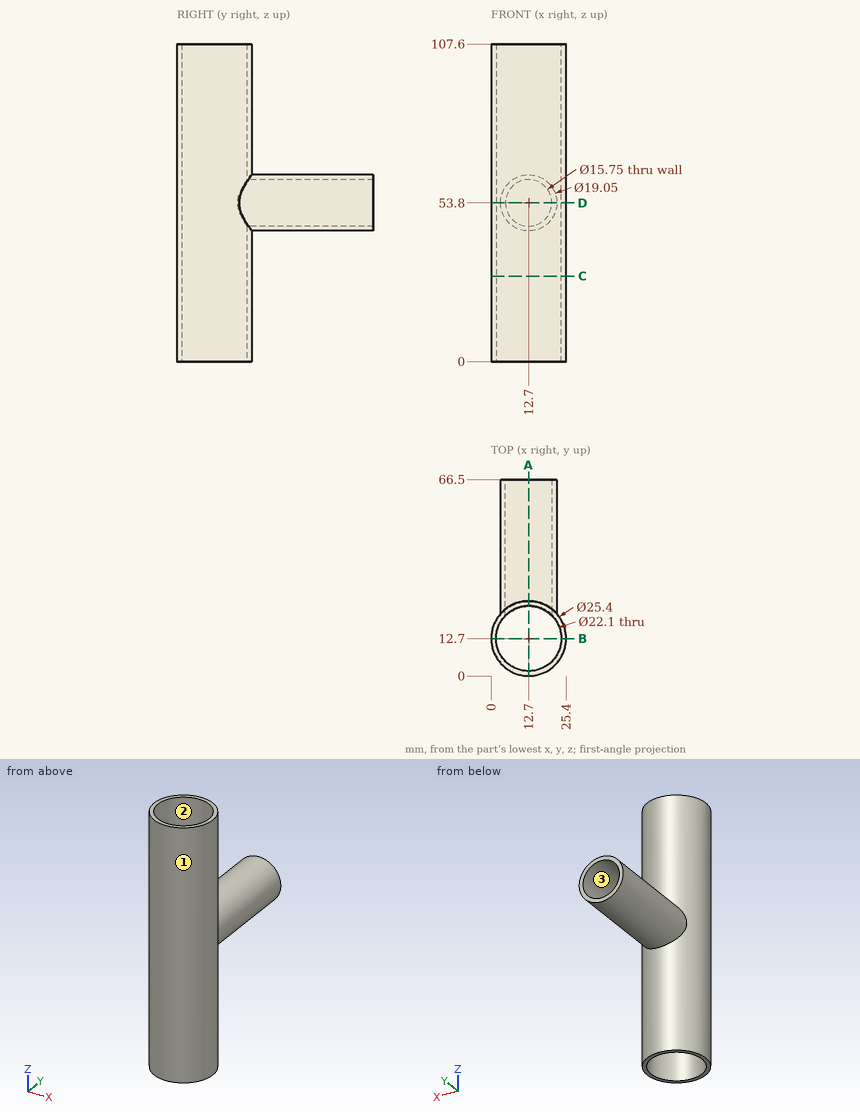
The figure shows three views and two pictorial views of one solid part (mm, origin at its lowest corner). Answer the questions. Give positions to 0.01 mm unless a question says otherwise; leave off trailing zeros. Loops run counter-clockwise (first coordinate to the right, second up) from the corner with the lowest first, then second, coordinate; pieces in that order, holes last. Notation, with made-up numbers: (-38.75, -6) -> (-25.75, -6) arc R23 cw to (-25.75, 20) -> close; hole circle Ø11 at (41.5, -37). An arc over 180 degrees is marked (long way). Use CSV: the item, a comma, the result in double quotes.
1. The part is cut by section B-B (y = 12.7). Write down the section's boundary in (x, z), then the cut area to 3 significant figures.
Found:
outline,"(0, 0) -> (1.65, 0) -> (1.65, 107.6) -> (0, 107.6) -> close; (23.75, 0) -> (25.4, 0) -> (25.4, 107.6) -> (23.75, 107.6) -> close"
area,"355 mm^2"
2. The part is cut by section A-A (x = 12.7). Write down the section's boundary in (y, z) (3 decimals), then the cut area to 3 significant figures.
Found:
outline,"(0, 0) -> (1.65, 0) -> (1.65, 107.6) -> (0, 107.6) -> close; (23.75, 0) -> (25.4, 0) -> (25.4, 44.275) -> (66.5, 44.275) -> (66.5, 45.925) -> (23.75, 45.925) -> close; (23.75, 61.675) -> (66.5, 61.675) -> (66.5, 63.325) -> (25.4, 63.325) -> (25.4, 107.6) -> (23.75, 107.6) -> close"
area,"465 mm^2"
3. Straight lines are drawn through the part: line 1 (Y direction, x = 12.7, z = 42.5); line 2 (Z direction, x = 12.7, y = 37) (3 decimals); line 3 (Y direction, x = 12.7, z = 48). For each, find the intervals that lie inside material, in ascending order.
Found:
line 1,"0 to 1.65, 23.75 to 25.4"
line 2,"44.275 to 45.925, 61.675 to 63.325"
line 3,"0 to 1.65"
4. Flat-ended cylindrical pins translate along their axes: pin 1 Ø1.5 at (x, z) = (21, 35.5) entering from +Y; pin 2 Ø12 at (x, y) = (19, 33.5) entering from +Z; pin 3 Ø3 at (x, z) = (5.5, 72) entering from -Y. Find the tip coordinate at first contact, or state that the pin passes through.
Found:
pin 1,"y = 22.91"
pin 2,"z = 63.32"
pin 3,"y = 1.35"
5. The mould has two halves that part along Y. Classify the marked faces 1, 2 and 3: +Y half, -Y half, draft (parallel to the pull), parting line (faces both ways), or undercut.
Found:
face 1,"parting line"
face 2,"undercut"
face 3,"draft"
6. The part is cut by section D-D (z = 53.8). Write down the section's boundary in (x, y) (3 decimals).
Found:
outline,"(3.175, 21.1) arc R12.7 ccw (long way) to (22.225, 21.1) -> (22.225, 66.5) -> (20.575, 66.5) -> (20.575, 20.452) arc R11.05 cw (long way) to (4.825, 20.452) -> (4.825, 66.5) -> (3.175, 66.5) -> close"
7. The part is cut by section C-C (z = 29). Write down the section's boundary in (x, y), then the cut area to 3 significant figures.
Found:
outline,"circle Ø25.4 at (12.7, 12.7); hole circle Ø22.1 at (12.7, 12.7)"
area,"123 mm^2"
